The listing builds one solid part. Answer for the finished solid, in the listing's coordinates (mm). Face numbers are marked on the shaded views. Round coordinates to 2 decimals unless told otherwise and drop trailing zeros. Write each loop counter-clockwise with the first axis right and the second up, starting at its lowest first coordinate (ties: lowest second). Pieces come first, ordered by that corner, then holes.
Item 1: Each of these flat-tipped pins is pushed along its axis until it touches: pin 1 (10 mm diameter, centred on x = 29.5, y = -22.5, fed in from +Z); pin 2 (4 mm diameter, centred on y = 13.5, z = 59, fed in from +X); pin 3 (8 mm diameter, centred on y = -24, z = 44.5, fed in from -X); pin 4 (4 mm diameter, centred on x = -6.5, y = -16, fed in from +Z) (3 decimals). Where does it stop, or does it pass through?
Item 2: Find section A-A on x = 37. Give the vertices of the cut face in (y, z).
Item 3: Find the intervals of material crossed by probe 1 along Y at (x, z) = (0, 89.5); probe 2 along Z at (x, y) = (30.5, 31.5); probe 3 along Y at (x, z) = (-8, 72.5), in increasing order.
Item 4: For a pull along Y with two mould halves and no side action, classify the marked faces 1 and 2 as +Y half, -Y half, draft (parallel to the pull), parting line (faces both ways), or undercut.
Item 5: Find section B-B on y = -39. Give the vertices of the cut face in (x, z), then the cut area to 3 significant figures.
Autodesk Fusion 360 part; units mm, degrees
sketch "Sketch1" plane through (0, 0, 0) normal (0, 0, 1) x (1, 0, 0)
  line L0 (-13.5, 19) -> (13.5, 19)
  line L1 (13.5, 19) -> (13.5, -19)
  line L2 (13.5, -19) -> (-13.5, -19)
  line L3 (-13.5, -19) -> (-13.5, 19)
  line L4 (-13.5, 19) -> (13.5, -19) construction
  line L5 (14.5, -20) -> (-14.5, -20)
  line L6 (-14.5, -20) -> (-14.5, 20)
  line L7 (-14.5, 20) -> (14.5, 20)
  line L8 (14.5, 20) -> (14.5, -20)
  line L9 (-45, 45) -> (45, 45)
  line L10 (45, 45) -> (45, -45)
  line L11 (45, -45) -> (-45, -45)
  line L12 (-45, -45) -> (-45, 45)
  line L13 (-45, 45) -> (45, -45) construction
  line L14 (-14.5, -20) -> (-45, -45)
  line L15 (-14.5, 20) -> (-45, 45)
  line L16 (14.5, 20) -> (45, 45)
  line L17 (14.5, -20) -> (45, -45)
  line L18 (-43.5, 43.5) -> (43.5, 43.5)
  line L19 (43.5, 43.5) -> (43.5, -43.5)
  line L20 (43.5, -43.5) -> (-43.5, -43.5)
  line L21 (-43.5, -43.5) -> (-43.5, 43.5)
  line L22 (-12.9225, 20) -> (-41.5925, 43.5)
  line L23 (-14.5, 18.707) -> (-43.5, 42.4775)
  line L24 (14.5, 18.707) -> (43.5, 42.4775)
  line L25 (12.9225, 20) -> (41.5925, 43.5)
  line L26 (12.9225, -20) -> (41.5925, -43.5)
  line L27 (14.5, -18.707) -> (43.5, -42.4775)
  line L28 (-14.5, -18.707) -> (-43.5, -42.4775)
  line L29 (-12.9225, -20) -> (-41.5925, -43.5)
  dimension "d5" = 27
  dimension "d6" = 38
  dimension "d15" = 90
  dimension "d16" = 90
  dimension "d44" = 1.5
ref_plane "WorkPlane1" through (0, 0, 85) normal (0, 0, 1) x (1, 0, 0)
sketch "Sketch2" plane through (0, 0, 85) normal (0, 0, 1) x (1, 0, 0)
  circle A0 centre (0, 0) radius 28.75
  circle A1 centre (0, 0) radius 30.5
  circle A2 centre (0, 0) radius 28.25
  circle A3 centre (0, 0) radius 31
  dimension "d10" = 57.5
  dimension "d11" = 61
  dimension "d13" = -0.5
  dimension "d14" = 0.5
loft "Loft3" add profiles "Sketch1", "Sketch2" section 1 contours L5 L6 L7 L8 section 2 contours A0 | A1 | A3 makes body 1
loft "Loft4" cut profiles "Sketch2", "Sketch1" section 1 contours A2 section 2 contours L0 L1 L2 L3 bodies 1
extrude "Extrude3" add sketch "Sketch1" along normal blind 1.5 separate body contours L5 L17 L20 L26 | L8 L17 L19 L20 L27 | L5 L20 L26 L29 | L8 L19 L24 L27 | L10 L16 L17 L18 L19 L20 | L11 L14 L17 L20 | L5 L14 L20 L29 | L8 L16 L18 L19 L24 | L6 L14 L20 L21 L28 | L7 L16 L18 L25 | L9 L15 L16 L18 | L12 L14 L15 L18 L20 L21 | L6 L21 L23 L28 | L7 L18 L22 L25 | L6 L15 L18 L21 L23 | L7 L15 L18 L22 makes body 2
extrude "Extrude4" add sketch "Sketch2" along normal blind 7 bodies 1
extrude "Extrude7" add sketch "Sketch1" along normal blind 3 contours L5 L17 L20 L26 | L8 L17 L19 L20 L27 | L10 L16 L17 L18 L19 L20 | L11 L14 L17 L20 | L5 L14 L20 L29 | L8 L16 L18 L19 L24 | L6 L14 L20 L21 L28 | L7 L16 L18 L25 | L9 L15 L16 L18 | L12 L14 L15 L18 L20 L21 | L6 L15 L18 L21 L23 | L7 L15 L18 L22 bodies 1 2
fillet "Fillet1" radius 3 4 edges at (45, -45, 1.5) (-45, -45, 1.5) (-45, 45, 1.5) (45, 45, 1.5) on bodies 1
equation "aparture_x = 27 mm"
equation "aparture_y = 38 mm"
equation "tube_height = 85 mm"
equation "wall_thickness = 1 mm"
equation "d5 = aparture_x"
equation "d6 = aparture_y"
equation "d7 = tube_height"
equation "hood_inner_dia = 57.5 mm"
equation "hood_outer_dia = 61 mm"
equation "d10 = hood_inner_dia"
equation "d11 = hood_outer_dia"
equation "d13 = -wall_thickness / 2"
equation "d14 = wall_thickness / 2"
equation "d15 = raft_y"
equation "d16 = raft_x"
equation "base_height = 1.5 mm"
equation "d22 = base_height"
equation "hood_lip_height = 7 mm"
equation "d25 = hood_lip_height"
equation "raft_x = 90 mm"
equation "raft_y = raft_x"
equation "rib_width = 1.5 mm"
equation "d44 = rib_width"
equation "rib_height = 1.5 mm"
equation "d54 = base_height + rib_height"
equation "round_corner_radius = 3 mm"
equation "d58 = round_corner_radius"
equation "tube_base_fillet_radius = 2 mm"
equation "d61 = tube_base_fillet_radius"
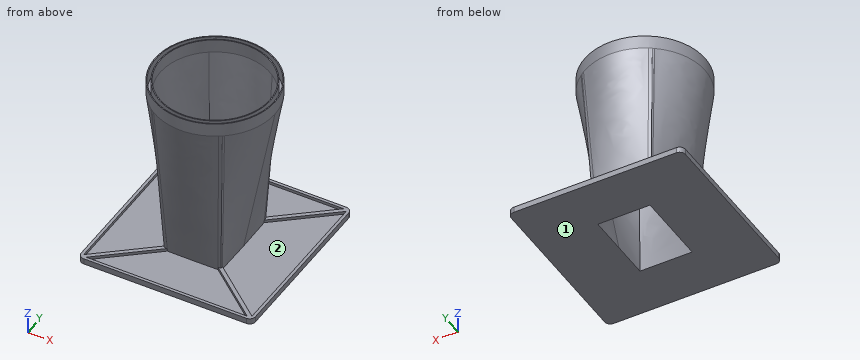
Check values:
1. pin 1: stops at z = 1.5
1. pin 2: stops at x = 24.14
1. pin 3: stops at x = -17.96
1. pin 4: passes through
2. outline: (-45, 0) - (45, 0) - (45, 3) - (43.5, 3) - (43.5, 1.5) - (39.74, 1.5) - (39.74, 3) - (37.15, 3) - (37.15, 1.5) - (-37.15, 1.5) - (-37.15, 3) - (-39.74, 3) - (-39.74, 1.5) - (-43.5, 1.5) - (-43.5, 3) - (-45, 3) - close
3. probe 1: y = -31 to -30.5, -28.75 to -28.25, 28.25 to 28.75, 30.5 to 31
3. probe 2: z = 0 to 1.5
3. probe 3: y = -28.41 to -25.84, 25.84 to 28.41
4. face 1: draft
4. face 2: undercut
5. outline: (-45, 0) - (45, 0) - (45, 3) - (43.5, 3) - (43.5, 1.5) - (39.26, 1.5) - (39.26, 3) - (36.1, 3) - (36.1, 1.5) - (-36.1, 1.5) - (-36.1, 3) - (-39.26, 3) - (-39.26, 1.5) - (-43.5, 1.5) - (-43.5, 3) - (-45, 3) - close
5. area: 149 mm2
